Read the model definition and answer for the solid it produces. Units are mm, in the model's axes. Coordinates: 2 decimals unless noted, no trailing zeros. Order: outer loops, then holes, each group sorted by start corner. A loop starts at its lowest first (then second) coordinate and runs counter-clockwise, first axis right, second up. Notation, with made-up numbers: (37, 1.5) - (44, 1.5) arc R24 cw to (44, 31.5) - close; hole circle Ø9 at (14.5, 38.5). An arc over 180 degrees is marked (long way). Use one line per item in the form item = value. Start each with the question number.
from build123d import *

# Parameters (mm, degrees)
SKETCH_W               = 20
SKETCH_H               = 19
PAD_DEPTH              = 2
SKETCH001_R            = 0.5
POCKET_DEPTH           = 5
LINEARPATTERN_COUNT    = 7
LINEARPATTERN_PITCH    = 2
SKETCH002_R            = 0.5
POCKET001_DEPTH        = 5
LINEARPATTERN001_COUNT = 8
LINEARPATTERN001_PITCH = 2


with BuildPart() as part:
    # Sketch → Pad (new body)
    with BuildSketch(Plane.XY):
        Rectangle(SKETCH_W, SKETCH_H)
    extrude(amount=PAD_DEPTH)

    # Sketch001 (on Face6 of Pad) → Pocket (cut)
    with BuildSketch(Plane.XY.offset(2)):
        with Locations((-8, 8.5)):
            Circle(SKETCH001_R)
        with Locations((8, 8.5)):
            Circle(SKETCH001_R)
    pocket = extrude(amount=-POCKET_DEPTH, mode=Mode.SUBTRACT)

    # LinearPattern: Pocket ×7
    with Locations(*[(0, -i * LINEARPATTERN_PITCH, 0) for i in range(1, LINEARPATTERN_COUNT)]):
        add(pocket, mode=Mode.SUBTRACT)

    # Sketch002 (on Face5 of LinearPattern) → Pocket001 (cut)
    with BuildSketch(Plane.XY.offset(2)):
        with Locations((-7, -7.5)):
            Circle(SKETCH002_R)
    pocket001 = extrude(amount=-POCKET001_DEPTH, mode=Mode.SUBTRACT)

    # LinearPattern001: Pocket001 ×8
    with Locations(*[(i * LINEARPATTERN001_PITCH, 0, 0) for i in range(1, LINEARPATTERN001_COUNT)]):
        add(pocket001, mode=Mode.SUBTRACT)


solid = part.part
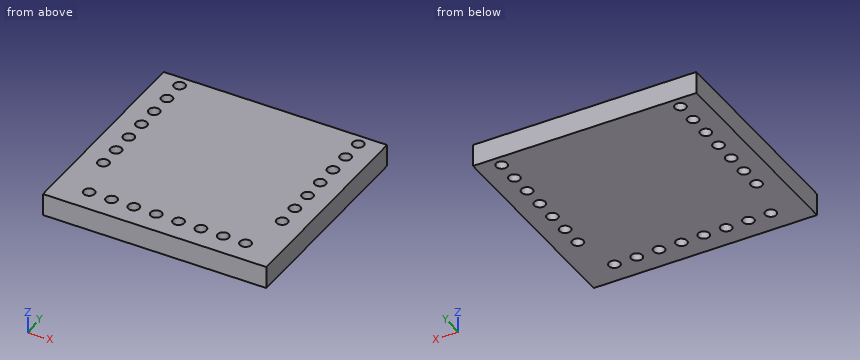
Q1. A cutting plane is placed at C-C (y = 4.5). Give the vertices of the cut face in (x, z), then the cut area to 3 significant figures.
Q2. A cutting plane is placed at A-A (z = 1.2). Give the number of separate pieces and of enclosed holes in the cut face, then the cut area to 3 significant figures.
Q3. Given P1, Ø8, axis at x = 1.5, y = 4.5, coming from the -Z side, flat-ended and moving along its own axis, determine where the tip first touches the part or whether it passes through.
Q4. Consider probe 1 along Y at (x, z) = (5, 0.6). Determine where the line is inside the solid, lowest interval first.
Q5. A cutting plane is placed at D-D (x = 1). Give the vertices of the cut face in (y, z).
Result sheet:
q1.outline = (-10, 0) - (-8.5, 0) - (-8.5, 2) - (-10, 2) - close; (-7.5, 0) - (7.5, 0) - (7.5, 2) - (-7.5, 2) - close; (8.5, 0) - (10, 0) - (10, 2) - (8.5, 2) - close
q1.area = 36.0 mm^2
q2.separate_pieces = 1
q2.enclosed_holes = 22
q2.area = 363 mm^2
q3.P1 = 0
q4.probe_1 = -9.5 to -8, -7 to 9.5
q5.outline = (-9.5, 0) - (-8, 0) - (-8, 2) - (-9.5, 2) - close; (-7, 0) - (9.5, 0) - (9.5, 2) - (-7, 2) - close
